Design review of the part shown in the three views and the two pictorial views. Dimensions are in mm from the part's minimum x, y and z. A direction names the side the tool comes from. Round coordinates to 2 decimals unless told otherwise and drop trailing zeros. Order: outer loops, then holes, each group sorted by start corner. A loop starts at its lowest first (then second) coordinate and runs counter-clockwise, first axis right, second up.
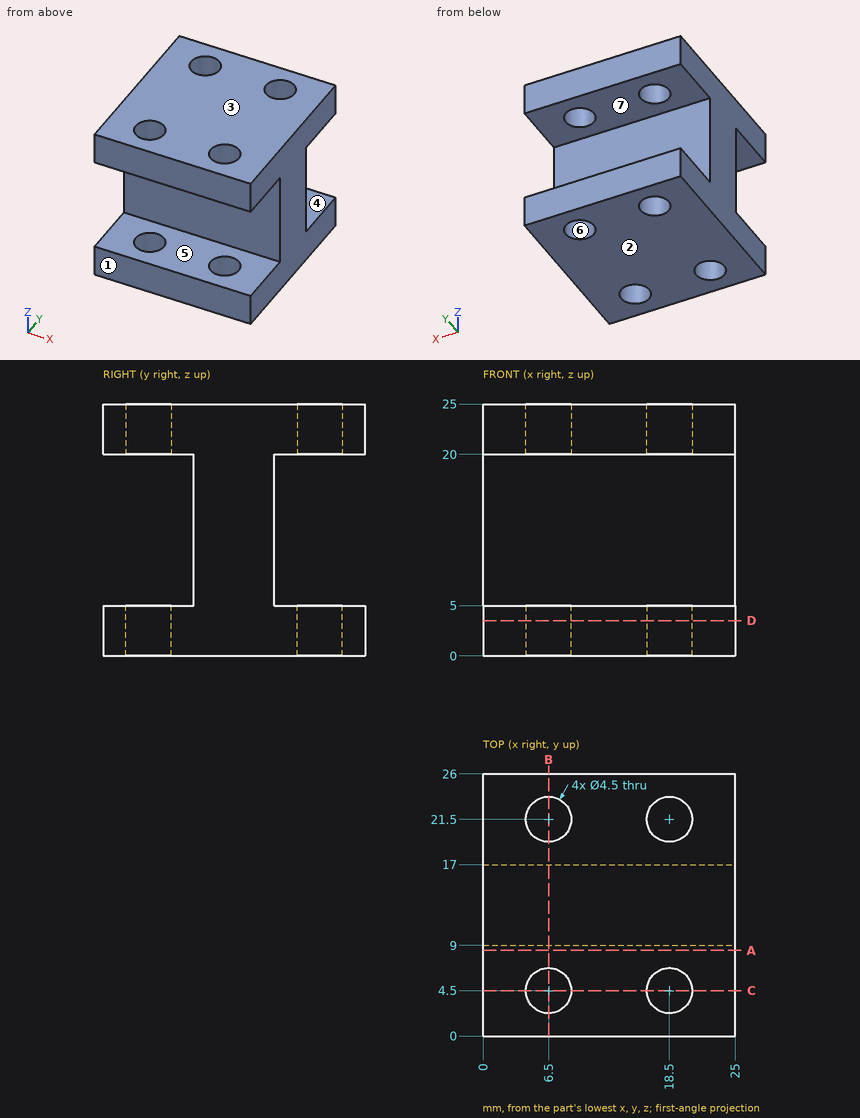
1) Clearance check with flat-ended pins moving along their axes: P1, Ø3.5, axis at x = 18.5, y = 4.5, coming from the +Z side; P2, Ø3, axis at x = 13.5, z = 7, coming from the -Y side; P3, Ø12, axis at x = 9.5, z = 13, coming from the +Y side. State where each tip first meets the part, or that it passes through.
Results:
P1: passes through
P2: stops at y = 9
P3: stops at y = 17
2) Take a section at B-B on x = 6.5. Give the boundary of the cut face in (y, z).
Results:
outline: (0, 0) - (2.25, 0) - (2.25, 5) - (0, 5) - close; (0, 20) - (2.25, 20) - (2.25, 25) - (0, 25) - close; (6.75, 0) - (19.25, 0) - (19.25, 5) - (17, 5) - (17, 20) - (19.25, 20) - (19.25, 25) - (6.75, 25) - (6.75, 20) - (9, 20) - (9, 5) - (6.75, 5) - close; (23.75, 0) - (26, 0) - (26, 5) - (23.75, 5) - close; (23.75, 20) - (26, 20) - (26, 25) - (23.75, 25) - close
3) For the marked faces 5, 6 and 7, list the 3-axis set-ups (+Z, -Z, +X, -X, +Y, -Y) from which the entire face can be reached by the end or side of a thin tool; tool diameter is ignored.
Results:
face 5: +X, -X, -Y
face 6: +Z, -Z
face 7: +X, -X, +Y
4) The part is to be moulded in two halves that separate along Z. For the marked faces 1, 2, 3 and 4, say which applies: released by +Z, released by -Z, zero draft, split by the parting line, or undercut.
Results:
face 1: zero draft
face 2: released by -Z
face 3: released by +Z
face 4: undercut
5) Take a section at A-A on y = 8.5. Give the boundary of the cut face in (x, z).
Results:
outline: (0, 0) - (25, 0) - (25, 5) - (0, 5) - close; (0, 20) - (25, 20) - (25, 25) - (0, 25) - close
6) To check wall thickness, follow line 1 along Y through (x, z) = (6.5, 23.6); line 2 along Z through (x, y) = (5.25, 7.5); line 3 along X through (y, z) = (20, 3). State the ranges of each line that lie inside material, in increasing order.
Results:
line 1: y = 0 to 2.25, 6.75 to 19.25, 23.75 to 26
line 2: z = 0 to 5, 20 to 25
line 3: x = 0 to 4.82, 8.18 to 16.82, 20.18 to 25
7) Take a section at C-C on y = 4.5. Give the boundary of the cut face in (x, z), plus the area to 3 significant figures.
Results:
outline: (0, 0) - (4.25, 0) - (4.25, 5) - (0, 5) - close; (0, 20) - (4.25, 20) - (4.25, 25) - (0, 25) - close; (8.75, 0) - (16.25, 0) - (16.25, 5) - (8.75, 5) - close; (8.75, 20) - (16.25, 20) - (16.25, 25) - (8.75, 25) - close; (20.75, 0) - (25, 0) - (25, 5) - (20.75, 5) - close; (20.75, 20) - (25, 20) - (25, 25) - (20.75, 25) - close
area: 160 mm2
8) Take a section at D-D on z = 3.5. Give the boundary of the cut face in (x, y), plus the area to 3 significant figures.
Results:
outline: (0, 0) - (25, 0) - (25, 26) - (0, 26) - close; hole circle Ø4.5 at (6.5, 4.5); hole circle Ø4.5 at (6.5, 21.5); hole circle Ø4.5 at (18.5, 4.5); hole circle Ø4.5 at (18.5, 21.5)
area: 586 mm2
